Check sheet for the modelled part. Datum: model origin and axes. Units: mm. A direction names the side the tool comes from. Round coordinates to 2 decimals unless told otherwise and drop trailing zeros. Answer in a Markdown table with one row per item.
```python
from build123d import *

# Parameters (mm, degrees)
EXTRUDE_1_DEPTH     = 100
SKETCH_2_R          = 1.75
CUT_EXTRUDE_1_DEPTH = 100
SKETCH_3_R          = 3
CUT_EXTRUDE_2_DEPTH = 4.5


with BuildPart() as part:
    # 草图1 → 凸台-拉伸1 (new body)
    with BuildSketch(Plane.XY):
        with BuildLine():
            Line((2.95, 4.5), (2.307669683, 4.5))
            ThreePointArc((2.307669683, 4.5), (2.194280341, 4.464750894), (2.120859728, 4.371428571))
            ThreePointArc((2.120859728, 4.371428571), (1.880846451, 3.985070843), (1.514285714, 3.715790517))
            ThreePointArc((1.514285714, 3.715790517), (1.430969149, 3.641993433), (1.4, 3.535088936))
            Line((1.4, 3.535088936), (1.4, 3.5))
            ThreePointArc((1.4, 3.5), (1, 3.1), (0.6, 3.5))
            Line((0.6, 3.5), (0.6, 3.535088936))
            ThreePointArc((0.6, 3.535088936), (0.569030851, 3.641993433), (0.485714286, 3.715790517))
            ThreePointArc((0.485714286, 3.715790517), (0.119153549, 3.985070843), (-0.120859728, 4.371428571))
            ThreePointArc((-0.120859728, 4.371428571), (-0.194280341, 4.464750894), (-0.307669683, 4.5))
            Line((-0.307669683, 4.5), (-2.65, 4.5))
            Line((-2.65, 4.5), (-3.25, 3.9))
            Line((-3.25, 3.9), (-3.25, -3.9))
            Line((-3.25, -3.9), (-2.65, -4.5))
            Line((-2.65, -4.5), (-0.307669683, -4.5))
            ThreePointArc((-0.307669683, -4.5), (-0.194280341, -4.464750894), (-0.120859728, -4.371428571))
            ThreePointArc((-0.120859728, -4.371428571), (0.119153549, -3.985070843), (0.485714286, -3.715790517))
            ThreePointArc((0.485714286, -3.715790517), (0.569030851, -3.641993433), (0.6, -3.535088936))
            Line((0.6, -3.535088936), (0.6, -3.5))
            ThreePointArc((0.6, -3.5), (1, -3.1), (1.4, -3.5))
            Line((1.4, -3.5), (1.4, -3.535088936))
            ThreePointArc((1.4, -3.535088936), (1.430969149, -3.641993433), (1.514285714, -3.715790517))
            ThreePointArc((1.514285714, -3.715790517), (1.880846451, -3.985070843), (2.120859728, -4.371428571))
            ThreePointArc((2.120859728, -4.371428571), (2.194280341, -4.464750894), (2.307669683, -4.5))
            Line((2.307669683, -4.5), (2.95, -4.5))
            ThreePointArc((2.95, -4.5), (3.162132034, -4.412132034), (3.25, -4.2))
            Line((3.25, -4.2), (3.25, 4.2))
            ThreePointArc((3.25, 4.2), (3.162132034, 4.412132034), (2.95, 4.5))
        make_face()
    extrude(amount=EXTRUDE_1_DEPTH)

    # 草图2 → 切除-拉伸1 (cut)
    with BuildSketch(Plane(origin=(3.25, 0, 0), x_dir=(0, 0, -1), z_dir=(1, 0, 0))):
        with Locations(Location((-6.386586206, 0, 0), (0, 0, 90))):
            Circle(SKETCH_2_R)
        with Locations(Location((-26.386586206, 0, 0), (0, 0, 90))):
            Circle(SKETCH_2_R)
        with Locations(Location((-46.386586206, 0, 0), (0, 0, 90))):
            Circle(SKETCH_2_R)
        with Locations(Location((-66.386586206, 0, 0), (0, 0, 90))):
            Circle(SKETCH_2_R)
        with Locations(Location((-86.386586206, 0, 0), (0, 0, 90))):
            Circle(SKETCH_2_R)
    extrude(amount=-CUT_EXTRUDE_1_DEPTH, mode=Mode.SUBTRACT)

    # 草图3 → 切除-拉伸2 (cut)
    with BuildSketch(Plane(origin=(3.25, 0, 0), x_dir=(0, 0, -1), z_dir=(1, 0, 0))):
        with Locations(Location((-6.386586206, 0, 0), (0, 0, 90))):
            Circle(SKETCH_3_R)
        with Locations(Location((-26.386586206, 0, 0), (0, 0, 90))):
            Circle(SKETCH_3_R)
        with Locations(Location((-46.386586206, 0, 0), (0, 0, 90))):
            Circle(SKETCH_3_R)
        with Locations(Location((-66.386586206, 0, 0), (0, 0, 90))):
            Circle(SKETCH_3_R)
        with Locations(Location((-86.386586206, 0, 0), (0, 0, 90))):
            Circle(SKETCH_3_R)
    extrude(amount=-CUT_EXTRUDE_2_DEPTH, mode=Mode.SUBTRACT)


solid = part.part
```
(1) Tool access check on faces 4 (the cylindrical face through (-2.24, -0.38, 4.68)), 5 (the cylindrical face through (1.031, -0.65, 63.458)). Record the directions out of +Z, -Z, +X, -X, +Y, -Y that give a thin tool (end or side, any length) a straight path to the whole face; none if there is none.
Solutions:
| item | result |
|---|---|
| face 4 | +X, -X |
| face 5 | +X |
(2) Scan lines: probe 1 along Z at (x, y) = (-2.8, 0); probe 2 along Z at (x, y) = (1.7, 0); probe 3 along Y at (x, z) = (2.5, 66.5). Record each from-to range of solid material in increasing order. Write a range as from..to.
Solutions:
| item | result |
|---|---|
| probe 1 | 0..4.64, 8.14..24.64, 28.14..44.64, 48.14..64.64, 68.14..84.64, 88.14..100 |
| probe 2 | 0..3.39, 9.39..23.39, 29.39..43.39, 49.39..63.39, 69.39..83.39, 89.39..100 |
| probe 3 | -4.5..-3, 3..4.5 |
(3) Depth check by flat-ended pin: pin 1 Ø3 at (y, z) = (0, 6.39) entering from +X; pin 2 Ø3 at (y, z) = (0, 7) entering from +X. Enter the tip coordinate at first touch or a pass-through.
Solutions:
| item | result |
|---|---|
| pin 1 | through |
| pin 2 | x = -1.25 |
(4) Draft check along Y on faces 1 (the flat face through (0, 0, 100)), 2 (the cylindrical face through (1.031, -0.65, 83.458)), 3 (the flat face through (-1, 4.5, 49)). Enter one of: pulls with the +Y half, pulls with the -Y half, needs draft (parallel to the pull), parting line crosses it, or undercut.
Solutions:
| item | result |
|---|---|
| face 1 | needs draft |
| face 2 | undercut |
| face 3 | pulls with the +Y half |
(5) Section check B-B on y = 0. Give the number of separate pieces and of enclosed holes in the cut face, plus the area to 3 significant figures.
Solutions:
| item | result |
|---|---|
| separate pieces | 6 |
| enclosed holes | 0 |
| area | 480 mm^2 |
